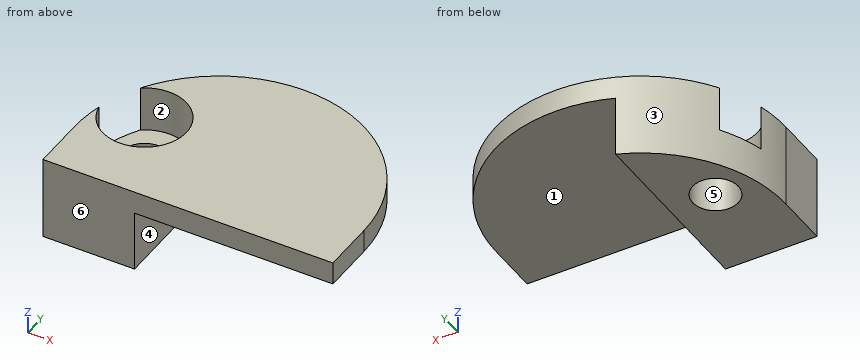
from build123d import *

# Parameters (mm, degrees)
ESBO_O1_R                = 1.5
RESSALTO_EXTRUS_O1_DEPTH = 5.5
ESBO_O2_W                = 13
ESBO_O2_H                = 14.546827215
CORTE_EXTRUS_O1_DEPTH    = 4
ESBO_O3_R                = 2.75
CORTE_EXTRUS_O2_DEPTH    = 3


with BuildPart() as part:
    # Esboço1 → Ressalto-extrusão1 (new body)
    with BuildSketch(Plane.XY):
        with BuildLine():
            Line((-9.5, 0), (-9.5, -3.5))
            Line((-9.5, -3.5), (9.5, -3.5))
            Line((9.5, -3.5), (9.5, 0))
            ThreePointArc((9.5, 0), (0, 9.5), (-9.5, 0))
        make_face()
        with Locations((-6.5, 2.75)):
            Circle(ESBO_O1_R, mode=Mode.SUBTRACT)
    extrude(amount=RESSALTO_EXTRUS_O1_DEPTH)

    # Esboço2 → Corte-extrusão1 (cut)
    with BuildSketch(Plane(origin=(0, 0, 0), x_dir=(-1, 0, 0), z_dir=(0, 0, -1))):
        with Locations((-3, 3.773413608)):
            Rectangle(ESBO_O2_W, ESBO_O2_H)
    extrude(amount=-CORTE_EXTRUS_O1_DEPTH, mode=Mode.SUBTRACT)

    # Esboço3 → Corte-extrusão2 (cut)
    with BuildSketch(Plane.XY.offset(5.5)):
        with Locations((-6.5, 2.75)):
            Circle(ESBO_O3_R)
    extrude(amount=-CORTE_EXTRUS_O2_DEPTH, mode=Mode.SUBTRACT)


solid = part.part
Part model, mm, in its own coordinate system. Face numbers are marked on the shaded views. A direction names the side the tool comes from. Coordinates: 2 decimals unless noted, no trailing zeros. Order: outer loops, then holes, each group sorted by start corner. A loop starts at its lowest first (then second) coordinate and runs counter-clockwise, first axis right, second up.
(1) Slice it at C-C, the plane x = -6.5. Write the cut outline in (y, z).
Check sheet entries:
outline: (-3.5, 0) - (1.25, 0) - (1.25, 2.5) - (0, 2.5) - (0, 5.5) - (-3.5, 5.5) - close; (4.25, 0) - (6.93, 0) - (6.93, 5.5) - (5.5, 5.5) - (5.5, 2.5) - (4.25, 2.5) - close
(2) Probe L1, parallel to Z at x = -7, y = 4.75; L2, parallel to Z at x = -1.75, y = 0; L3, parallel to Y at x = -6.5, z = 3.85. List the from-to ranges inside material, lowest first.
Check sheet entries:
L1: z = 0 to 2.5
L2: z = 4 to 5.5
L3: y = -3.5 to 0, 5.5 to 6.93
(3) Slice it at A-A, the plane z = 0.6. Write the cut outline in (x, y), and give its area (3 significant figures).
Check sheet entries:
outline: (-9.5, -3.5) - (-3.5, -3.5) - (-3.5, 8.83) arc R9.5 ccw to (-9.5, 0) - close; hole circle Ø3 at (-6.5, 2.75)
area: 52.3 mm2
(4) Tool access for the marked faces 1, 2 and 3: list every direction of +Z, -Z, +X, -X, +Y, -Y with a clear straight run to the whole face (end or side of a thin tool).
Check sheet entries:
face 1: -Z, +X, +Y, -Y
face 2: +Z
face 3: +Z, -Z, +Y
(5) Slice it at D-D, the plane x = 0. Write the cut outline in (y, z), and give its area (3 significant figures).
Check sheet entries:
outline: (-3.5, 4) - (9.5, 4) - (9.5, 5.5) - (-3.5, 5.5) - close
area: 19.5 mm2
(6) Pin check, flat tips, straight feed: pin 1 Ø2 at (y, z) = (1.5, 4.5) entering from -X; pin 2 Ø4 at (x, y) = (5.5, 5.5) entering from -Z; pin 3 Ø2 at (y, z) = (5, 4.5) entering from +X; pin 4 Ø2.5 at (x, y) = (-6.5, 2.75) entering from -Z. Stop position of each tip, or through.
Check sheet entries:
pin 1: stops at x = -9.49
pin 2: stops at z = 4
pin 3: stops at x = 8.62
pin 4: passes through
(7) Pull direction Y, two halves, no side cores. Call the marked faces 4, 5 and 6: pulls with the +Y half, pulls with the -Y half, needs draft (parallel to the pull), parting line crosses it, or undercut.
Check sheet entries:
face 4: needs draft
face 5: undercut
face 6: pulls with the -Y half
(8) Slice it at B-B, the plane y = 1.75. Write the cut outline in (x, z), and give its area (3 significant figures).
Check sheet entries:
outline: (-9.34, 0) - (-7.62, 0) - (-7.62, 2.5) - (-9.06, 2.5) - (-9.06, 5.5) - (-9.34, 5.5) - close; (-5.38, 0) - (-3.5, 0) - (-3.5, 4) - (9.34, 4) - (9.34, 5.5) - (-3.94, 5.5) - (-3.94, 2.5) - (-5.38, 2.5) - close
area: 30.4 mm2
